```python
from build123d import *

# Parameters (mm, degrees)
BOSS_EXTRUDE1_DEPTH    = 72
SKETCH2_W              = 72
SKETCH2_H              = 6
CUT_EXTRUDE1_DEPTH     = 50
SKETCH3_R              = 30
CUT_EXTRUDE2_DEPTH     = 12
F_20_0MM_DOWEL_HOLE1_D = 24
CUT_EXTRUDE3_REACH     = 176.453


with BuildPart() as part:
    # Sketch1 → Boss-Extrude1 (new body)
    with BuildSketch(Plane.XY):
        Polygon((0, 66), (12, 66), (12, 20), (0, 20), (0, 0), (29.646636928, 0), (145, 0), (145, 25), (36, 25), (36, 90), (0, 90), align=None)
    extrude(amount=BOSS_EXTRUDE1_DEPTH)

    # Sketch2 → Cut-Extrude1 (cut)
    with BuildSketch(Plane.XY.offset(72)):
        with Locations((36, 3)):
            Rectangle(SKETCH2_W, SKETCH2_H)
    extrude(amount=-CUT_EXTRUDE1_DEPTH, mode=Mode.SUBTRACT)

    # Sketch3 → Cut-Extrude2 (cut)
    with BuildSketch(Plane.ZY.offset(-12)):
        with Locations((36, 43)):
            Circle(SKETCH3_R)
    extrude(amount=CUT_EXTRUDE2_DEPTH, mode=Mode.SUBTRACT)

    # Ø20.0mm Dowel Hole1 (through all)
    with Locations(Plane.ZY.offset(-12)):
        with Locations((36, 43)):
            Hole(F_20_0MM_DOWEL_HOLE1_D / 2)

    # Sketch8 → Cut-Extrude3 (cut, up to next)
    with BuildSketch(Plane(origin=(0, 25, 0), x_dir=(1, 0, 0), z_dir=(0, 1, 0)), mode=Mode.PRIVATE) as cut_extrude3_sk1:
        with BuildLine():
            Line((195, -48), (95, -48))
            ThreePointArc((95, -48), (83, -36), (95, -24))
            Line((95, -24), (195, -24))
            ThreePointArc((195, -24), (207, -36), (195, -48))
        make_face()
    cut_extrude3_tool1 = extrude(cut_extrude3_sk1.sketch, amount=-CUT_EXTRUDE3_REACH, mode=Mode.PRIVATE) & part.part
    add(cut_extrude3_tool1.solids().sort_by_distance((145, 25, 36))[0], mode=Mode.SUBTRACT)


solid = part.part
```
Source: CAD feature listing. Evaluate the final solid. Frame: model axes, mm. A direction names the side the tool comes from. Give positions to 0.01 mm unless a question says otherwise; leave off trailing zeros. Loops run counter-clockwise (first coordinate to the right, second up) from the corner with the lowest first, then second, coordinate; pieces in that order, holes last. Notation, with made-up numbers: (1.25, 54.25) -> (43.25, 54.25) arc R19 ccw to (43.25, 86.25) -> close; hole circle Ø2 at (30.25, 36). An arc over 180 degrees is marked (long way). Use a Markdown table: item, result. Add a question column.
(1) Ray query, line 1 (Y direction, x = 17.5, z = 36); line 2 (Z direction, x = 124, y = 14); line 3 (X direction, y = 67.5, z = 8.5). Return the intervals inside material, ascending.
(2) First-contact query: pin 1 Ø10 at (x, z) = (56.5, 48.5) entering from -Y; pin 2 Ø3 at (x, z) = (48, 30) entering from +Y; pin 3 Ø8 at (x, y) = (127, 30.5) entering from -Z; pin 4 Ø19.5 at (y, z) = (42, 38.5) entering from +X. Flat tips, straight axial feed; report the tip coordinate or a pass-through.
(3) Section query D-D (z = 63). Output: boundary loops of the cut face in (x, y).
(4) Section query C-C (z = 36). Output: boundary loops of the cut face in (x, y), then the cut area to 3 significant figures.
(5) Access query for faces 1 (the face through (35, 3, 22)), 2 (the face through (6, 20, 8)), 3 (the face through (6, 73, 36)), 4 (the face through (120, 13, 48)). Directions: +Z, -Z, +X, -X, +Y, -Y. A direction counts if a zero-diameter tool reaches every point of the face in a straight line with its end or side. Return the directions, or none.
(6) Section query A-A (x = 118.5). Output: boundary loops of the cut face in (y, z), then the cut area to 3 significant figures.
(7) Section query B-B (y = 43). Output: boundary loops of the cut face in (x, z).
(8) Pull-direction query (Y, two-part tool) for faces 5 (the face through (79, 25, 35)), 6 (the face through (12, 57, 35)), 7 (the face through (36, 57, 35)); classes: +Y half, -Y half, draft (parallel to the pull), parting line (faces both ways), or undercut.
Checked values:
| question | item | result |
|---|---|---|
| 1 | line 1 | 6 to 31, 55 to 90 |
| 1 | line 2 | 0 to 24, 48 to 72 |
| 1 | line 3 | 0 to 36 |
| 2 | pin 1 | y = 6 |
| 2 | pin 2 | y = 25 |
| 2 | pin 3 | through |
| 2 | pin 4 | x = 36 |
| 3 | outline | (0, 6) -> (72, 6) -> (72, 0) -> (145, 0) -> (145, 25) -> (36, 25) -> (36, 90) -> (0, 90) -> (0, 66) -> (12, 66) -> (12, 20) -> (0, 20) -> close |
| 4 | outline | (0, 6) -> (72, 6) -> (72, 0) -> (83, 0) -> (83, 25) -> (36, 25) -> (36, 31) -> (12, 31) -> (12, 13) -> (0, 13) -> close; (0, 73) -> (12, 73) -> (12, 55) -> (36, 55) -> (36, 90) -> (0, 90) -> close |
| 4 | area | 2,690 mm^2 |
| 5 | face 1 | +Z, -X, -Y |
| 5 | face 2 | +Z, -Z, -X |
| 5 | face 3 | -X |
| 5 | face 4 | +X, +Y, -Y |
| 6 | outline | (0, 0) -> (25, 0) -> (25, 24) -> (0, 24) -> close; (0, 48) -> (25, 48) -> (25, 72) -> (0, 72) -> close |
| 6 | area | 1,200 mm^2 |
| 7 | outline | (12, 0) -> (36, 0) -> (36, 24) -> (12, 24) -> close; (12, 48) -> (36, 48) -> (36, 72) -> (12, 72) -> close |
| 8 | face 5 | +Y half |
| 8 | face 6 | undercut |
| 8 | face 7 | draft |
